The model under review builds one solid part; all positions refer to its coordinate system, in mm. A direction names the side the tool comes from. Coordinates: 2 decimals unless noted, no trailing zeros. Order: outer loops, then holes, each group sorted by start corner. A loop starts at its lowest first (then second) coordinate and runs counter-clockwise, first axis right, second up. Notation, with made-up numbers: (-17.5, -14.75) -> (40.5, -14.75) arc R32 cw to (40.5, 19.25) -> close; hole circle Ø11 at (8.25, 48). An arc over 180 degrees is marked (long way). Answer as CSV lines item,"result". Start each with the question number.
from build123d import *

# Parameters (mm, degrees)
RESSALTO_EXTRUS_O1_DEPTH = 3
ESBO_O5_R                = 5
RESSALTO_EXTRUS_O2_DEPTH = 0.6


with BuildPart() as part:
    # Esboço4 → Ressalto-extrusão1 (new body)
    with BuildSketch(Plane.XY):
        with BuildLine():
            Line((-22, 0), (-22, 20.5))
            ThreePointArc((-22, 20.5), (-21.560660172, 21.560660173), (-20.499999999, 22.000000002))
            Line((-20.499999999, 22.000000002), (1e-09, 22.000000002))
            Line((1e-09, 22.000000002), (20.500000001, 22.000000002))
            ThreePointArc((20.500000001, 22.000000002), (21.560660174, 21.560660173), (22.000000003, 20.5))
            Line((22.000000003, 20.5), (22.000000003, 0))
            Line((22.000000003, 0), (22.000000003, -20.5))
            ThreePointArc((22.000000003, -20.5), (21.560660175, -21.560660173), (20.500000002, -22.000000002))
            Line((20.500000002, -22.000000002), (1e-09, -22.000000002))
            Line((1e-09, -22.000000002), (-20.499999999, -22.000000002))
            ThreePointArc((-20.499999999, -22.000000002), (-21.560660172, -21.560660173), (-22, -20.5))
            Line((-22, -20.5), (-22, 0))
        make_face()
    extrude(amount=RESSALTO_EXTRUS_O1_DEPTH)

    # Esboço5 → Ressalto-extrusão2 (add)
    with BuildSketch(Plane.XY.offset(3)):
        Circle(ESBO_O5_R)
    extrude(amount=RESSALTO_EXTRUS_O2_DEPTH)


solid = part.part
1) Tool access review of faces 1 (the face through (-1.08, -4.88, 3.3)), 2 (the face through (0, 0, 3.6)): name each direction out of +Z, -Z, +X, -X, +Y, -Y from which nothing blocks a thin tool from reaching the whole face with its end or side.
2) Wall thickness on L1, parallel to Z at x = 0.5, y = 7: over which ranges is the line inside the solid? List them lowest first. Write a range as [from, to].
3) Consider section A-A (y = 0). Give the boundary of the cut face in (x, z).
4) Consider section C-C (x = 12). Give the boundary of the cut face in (y, z).
5) Insertion check: pin 1 Ø6 at (x, y) = (-4, 3.5) entering from -Z; pin 2 Ø1.5 at (x, y) = (6.5, -9.5) entering from +Z. Each pin has a flat end and moves straight along its axis. Give the tip position at first contact, or say it passes through.
Result:
1,face 1,"+Z"
1,face 2,"+Z, +X, -X, +Y, -Y"
2,L1,"[0, 3]"
3,outline,"(-22, 0) -> (22, 0) -> (22, 3) -> (5, 3) -> (5, 3.6) -> (-5, 3.6) -> (-5, 3) -> (-22, 3) -> close"
4,outline,"(-22, 0) -> (22, 0) -> (22, 3) -> (-22, 3) -> close"
5,pin 1,"z = 0"
5,pin 2,"z = 3"
